```python
from build123d import *

# Parameters (mm, degrees)
SKETCH_1_R      = 2
SKETCH_1_R_2    = 1
EXTRUDE_1_DEPTH = 20
CHAMFER_1_SIZE  = 0.2


with BuildPart() as part:
    # Эскиз1 → Бобышка-Вытянуть1 (new body)
    with BuildSketch(Plane.XY):
        Circle(SKETCH_1_R)
        Circle(SKETCH_1_R_2, mode=Mode.SUBTRACT)
    extrude(amount=EXTRUDE_1_DEPTH)

    # Фаска1
    chamfer_1_edges = [part.edges().sort_by_distance(p)[0] for p in [
        (-2, 0, 0),
        (-2, 0, 20),
        (-1, 0, 0),
        (-1, 0, 20),
    ]]
    chamfer(chamfer_1_edges, length=CHAMFER_1_SIZE)


solid = part.part
```
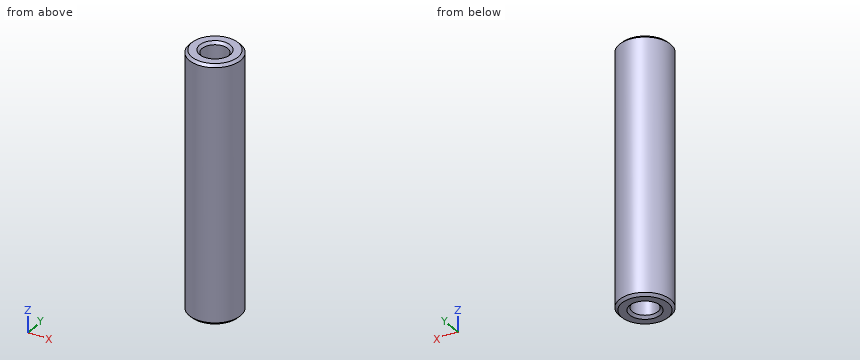
The model under review builds one solid part; all positions refer to its coordinate system, in mm. Give positions to 0.01 mm unless a question says otherwise; leave off trailing zeros. Write each loop counter-clockwise with the first axis right and the second up, starting at its lowest first coordinate (ties: lowest second). Pieces come first, ordered by that corner, then holes. Notation, with made-up numbers: M 55,85.25 L 77,85.25 A15 cw 77,110.25 Z; hole C -9.5,55.5 d6. An arc over 180 degrees is marked long. Write each question's results on one line, items separated by ' | '. Start each with the question number.
1. We need section A-A (x = 0). Write out the cut boundary in (y, z).
2. We need section C-C (z = 2.75). Write out the cut boundary in (x, y).
3. For probe 1 along X at (y, z) = (-0.05, 13); probe 2 along X at (y, z) = (0.75, 17), list the stretches that pass through material, from the lowest coordinate up. Write a range as [from, to].
Results found:
1) outline: M -2,0.2 L -1.8,0 L -1.2,0 L -1,0.2 L -1,19.8 L -1.2,20 L -1.8,20 L -2,19.8 Z; M 1,0.2 L 1.2,0 L 1.8,0 L 2,0.2 L 2,19.8 L 1.8,20 L 1.2,20 L 1,19.8 Z
2) outline: C 0,0 d4; hole C 0,0 d2
3) probe 1: x = [-2, -1], [1, 2] | probe 2: x = [-1.85, -0.66], [0.66, 1.85]
